Source: CAD feature listing. Evaluate the final solid. Frame: model axes, mm. Face numbers are marked on the shaded views. A direction names the side the tool comes from. Round coordinates to 2 decimals unless told otherwise and drop trailing zeros. Order: outer loops, then holes, each group sorted by start corner. A loop starts at its lowest first (then second) coordinate and runs counter-clockwise, first axis right, second up. Notation, with made-up numbers: (76, 43.25) - (114, 43.25) arc R24 ccw to (114, 75.25) - close; hole circle Ø3 at (7, -15). An arc over 180 degrees is marked (long way). Return JSON: item names as keys, results as strings. Group by question number.
1) Ray query, line 1 (Y direction, x = 0.15, z = 4). Return the intervals inside material, ascending. Write a range as from..to.
2) Section B-B, the plane z = 3. Return loops of the section in (x, y).
3) Contact query for flat-ended pins moving along their axis: P1, Ø0.9, axis at x = 2, y = -22.5, coming from the +Z side; P2, Ø1.5, axis at x = 1, z = 3, coming from the +Y side. Output: stop coordinate, or through.
4) Section A-A, the plane x = 1.8. Return loops of the section in (y, z), plus the area to 3 significant figures.
5) Access query for the marked faces 1 and 2. Directions: +Z, -Z, +X, -X, +Y, -Y. A direction counts if a zero-diameter tool reaches every point of the face in a straight line with its end or side. Return the directions, or none.
Autodesk Inventor part; units mm, degrees
ref_plane "YZ Plane" through (0, 0, 0) normal (1, 0, 0) x (0, 1, 0)
ref_plane "XZ Plane" through (0, 0, 0) normal (0, 1, 0) x (-1, 0, 0)
ref_plane "XY Plane" through (0, 0, 0) normal (0, 0, 1) x (1, 0, 0)
sketch "Boceto1" plane through (0, 0, 0) normal (1, 0, 0) x (0, 1, 0)
  line L0 (21.5, 1.5) -> (21.5, 4.5)
  line L1 (24.5, 1.5) -> (21.5, 1.5)
  line L2 (24.5, -4.5) -> (24.5, 1.5)
  line L3 (21.5, -4.5) -> (24.5, -4.5)
  line L4 (-21.5, -4.5) -> (21.5, -4.5)
  line L5 (-24.5, -4.5) -> (-21.5, -4.5)
  line L6 (-24.5, 1.5) -> (-24.5, -4.5)
  line L7 (-21.5, 1.5) -> (-24.5, 1.5)
  line L8 (-21.5, 4.5) -> (-21.5, 1.5)
  line L9 (21.5, 4.5) -> (-21.5, 4.5)
  point P0 (0, 0)
extrude "Extrusión1" add sketch "Boceto1" along normal blind 3
properties part number "Case_Base3" material "MDF Tablero de fibras de densidad media"
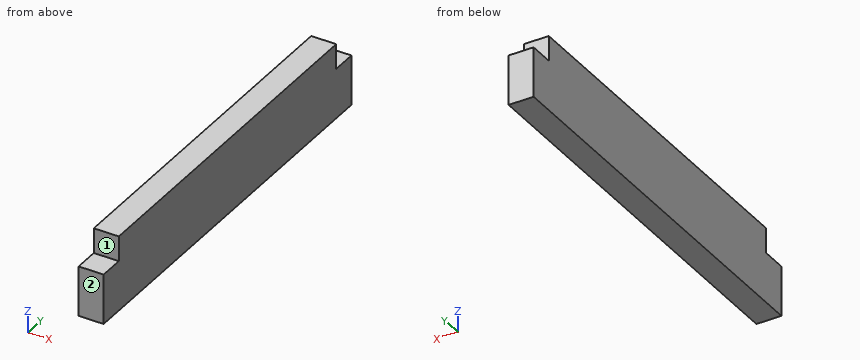
Geometry check:
{
 "1": {"line 1": "-21.5..21.5"},
 "2": {"outline": "(0, -21.5) - (3, -21.5) - (3, 21.5) - (0, 21.5) - close"},
 "3": {"P1": "z = 1.5", "P2": "y = 21.5"},
 "4": {"outline": "(-24.5, -4.5) - (24.5, -4.5) - (24.5, 1.5) - (21.5, 1.5) - (21.5, 4.5) - (-21.5, 4.5) - (-21.5, 1.5) - (-24.5, 1.5) - close", "area": "423 mm2"},
 "5": {"face 1": "+Z, +X, -X, -Y", "face 2": "+Z, -Z, +X, -X, -Y"}
}
